Source: CAD feature listing. Evaluate the final solid. Frame: model axes, mm. Face numbers are marked on the shaded views. Give positions to 0.01 mm unless a question says otherwise; leave off trailing zeros. Order: outer loops, then holes, each group sorted by start corner. A loop starts at its lowest first (then second) coordinate and runs counter-clockwise, first axis right, second up. Notation, with made-up numbers: M -14,79.5 L 32,79.5 A19 cw 32,115.5 Z; hole C 56,60.25 d4. An arc over 180 degrees is marked long. Answer in a Markdown table with one row per item. Add a question column.
(1) Section query C-C, the plane z = 55.5. Count the separate pieces of the cut face and the enclosed holes in it, plus the area to 3 significant figures.
(2) Section query D-D, the plane x = -132. Return loops of the section in (y, z).
(3) Section query A-A, the plane y = 0. Return loops of the section in (x, z), plus the area to 3 significant figures.
(4) Material intervals for line 1 along X through (y, z) = (-115.5, 40) (3 decimals); line 2 along Y through (x, z) = (1, 27); line 3 along X through (y, z) = (336.5, 46.5), sorted ascending.
(5) Pin query (flat end, axial travel): P1, Ø4, axis at x = 120.5, z = 29, coming from the -Y side; P2, Ø3, axis at x = 331.5, z = 23.5, coming from the +Y side; P3, Ø1.5, axis at x = 152, z = 19.5, coming from the -Y side. Return the tip coordinate at first contact, or that it passes through.
(6) Mould query, pull axis Y, two halves, no side actions, for the marked faces 1, 2 and 3. Classes: pulls with the +Y half, pulls with the -Y half, needs draft (parallel to the pull), parting line crosses it, or undercut.
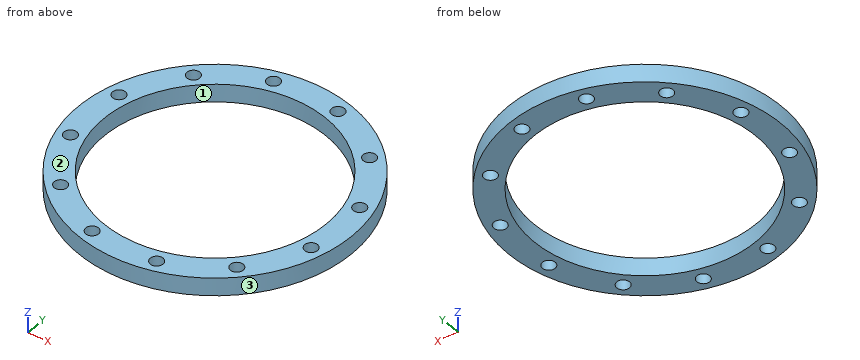
from build123d import *

# Parameters (mm, degrees)
SKETCH1_R               = 535
SKETCH1_R_2             = 435
BOSS_EXTRUDE1_DEPTH     = 70
CUT_EXTRUDE2_DEPTH      = 760.835508515
CUT_EXTRUDE2_DEPTH_BACK = 760.835508515
SKETCH3_R               = 25


with BuildPart() as part:
    # Sketch1 → Boss-Extrude1 (new body)
    with BuildSketch(Plane.XY):
        Circle(SKETCH1_R)
        Circle(SKETCH1_R_2, mode=Mode.SUBTRACT)
    extrude(amount=BOSS_EXTRUDE1_DEPTH)

    # Sketch3 → Cut-Extrude2 (cut, two sides: drawn at the far end of the back side and taken through both)
    with BuildSketch(Plane.XY.offset(70).offset(-CUT_EXTRUDE2_DEPTH_BACK)):
        with Locations((125.527236875, 468.47402575)):
            Circle(SKETCH3_R)
        with Locations((342.946788875, 342.946788875)):
            Circle(SKETCH3_R)
        with Locations((468.47402575, 125.527236875)):
            Circle(SKETCH3_R)
        with Locations((468.47402575, -125.527236875)):
            Circle(SKETCH3_R)
        with Locations((342.946788875, -342.946788876)):
            Circle(SKETCH3_R)
        with Locations((125.527236875, -468.47402575)):
            Circle(SKETCH3_R)
        with Locations((-125.527236875, -468.47402575)):
            Circle(SKETCH3_R)
        with Locations((-342.946788876, -342.946788875)):
            Circle(SKETCH3_R)
        with Locations((-468.47402575, -125.527236875)):
            Circle(SKETCH3_R)
        with Locations((-468.47402575, 125.527236875)):
            Circle(SKETCH3_R)
        with Locations((-342.946788875, 342.946788876)):
            Circle(SKETCH3_R)
        with Locations((-125.527236875, 468.47402575)):
            Circle(SKETCH3_R)
    extrude(amount=CUT_EXTRUDE2_DEPTH + CUT_EXTRUDE2_DEPTH_BACK, mode=Mode.SUBTRACT)


solid = part.part
Values follow:
| question | item | result |
|---|---|---|
| 1 | separate pieces | 1 |
| 1 | enclosed holes | 13 |
| 1 | area | 281,000 mm² |
| 2 | outline | M -518.46,0 L -492.62,0 L -492.62,70 L -518.46,70 Z; M -444.33,0 L -414.49,0 L -414.49,70 L -444.33,70 Z; M 414.49,0 L 444.33,0 L 444.33,70 L 414.49,70 Z; M 492.62,0 L 518.46,0 L 518.46,70 L 492.62,70 Z |
| 3 | outline | M -535,0 L -435,0 L -435,70 L -535,70 Z; M 435,0 L 535,0 L 535,70 L 435,70 Z |
| 3 | area | 14,000 mm² |
| 4 | line 1 | x = -522.384 to -491.375, -445.573 to -419.386, 419.386 to 445.573, 491.375 to 522.384 |
| 4 | line 2 | y = -535 to -435, 435 to 535 |
| 4 | line 3 | x = -415.92 to -367.1, -318.79 to -275.67, 275.67 to 318.79, 367.1 to 415.92 |
| 5 | P1 | stops at y = -521.71 |
| 5 | P2 | stops at y = 421.1 |
| 5 | P3 | stops at y = -513.17 |
| 6 | face 1 | undercut |
| 6 | face 2 | needs draft |
| 6 | face 3 | parting line crosses it |
